Work out the finished part from the listing and answer in its coordinate system (mm). Face numbers are marked on the shaded views. A direction names the side the tool comes from. Coordinates: 2 decimals unless noted, no trailing zeros. Write each loop counter-clockwise with the first axis right and the second up, starting at its lowest first coordinate (ties: lowest second). Pieces come first, ordered by that corner, then holes. Notation, with made-up numbers: M 17.25,73.5 L 76.25,73.5 A8 ccw 76.25,85.5 Z; hole C 80,-20 d11. An arc over 180 degrees is marked long. Answer as CSV lines item,"result". Start each with the question number.
(1) A cutting plane is placed at A-A on y = 28.5. Give the vertices of the cut face in (x, z), then the cut area to 3 significant figures.
(2) Flat-ended cylindrical pins translate along their axes: P1, Ø10, axis at x = -3.5, y = 26.5, coming from the +Z side; P2, Ø10, axis at x = 5, y = 10.5, coming from the -Z side; P3, Ø5, axis at x = 2, y = 31, coming from the -Z side. Find the tip coordinate at first contact, or state that the pin passes through.
(3) The mould has two halves that part along X. Classify the marked faces 1 and 2: released by +X, released by -X, zero draft, split by the parting line, or undercut.
(4) Find the intervals of material crossed by L1, parallel to Y at x = 7, z = -0.5; L2, parallel to Y at x = 5, z = -4.75; L3, parallel to Y at x = -8.5, z = -1.25, in increasing order. Write a range as [from, to].
(5) A cutting plane is placed at B-B on z = -9.5. Give the vertices of the cut face in (x, y), then the cut area to 3 significant figures.
(6) A cutting plane is placed at C-C on y = 8.5. Give the vertices of the cut face in (x, z), then the cut area to 3 significant figures.
(7) For the marked faces 3, 4 and 5, determine the directions among +Z, -Z, +X, -X, +Y, -Y from which every point of the face is accessible in a straight line to the end or side of a thin tool.
from build123d import *
from build123d.topology import SkipClean

# Parameters (mm, degrees)
SKETCH1_R           = 7.5
BOSS_EXTRUDE1_DEPTH = 20
CUT_EXTRUDE2_DEPTH  = 12
CUT_EXTRUDE4_DEPTH  = 1
CHAMFER1_SIZE       = 1
CHAMFER3_SIZE       = 2
CHAMFER4_SIZE       = 1


with BuildPart() as part:
    # Sketch1 → Boss-Extrude1 (new body)
    with BuildSketch(Plane(origin=(0, 0, 0), x_dir=(1, 0, 0), z_dir=(0, 1, 0))):
        with Locations(Location((0, 0, 0), (0, 0, 270))):
            Circle(SKETCH1_R)
    extrude(amount=BOSS_EXTRUDE1_DEPTH)

    # Sketch2 → Revolve1 (revolve)
    with BuildSketch(Plane.XY):
        with BuildLine():
            Line((7.5, 18.99999999999999), (7.5, 20))
            Line((7.5, 20), (0, 20))
            Line((0, 20), (3.1e-16, 39))
            Line((3.1e-16, 39), (7.500000000000009, 39))
            ThreePointArc((7.500000000000009, 39), (12.500000000000009, 28.999999999999993), (7.5, 18.99999999999999))
        make_face()
    revolve(axis=Axis((0, 20, 0), (2e-17, 1, 0)))

    # Sketch3 → Cut-Extrude2 (cut)
    with BuildSketch(Plane(origin=(0, 0, 0), x_dir=(-1, 0, 0), z_dir=(0, -1, 0))):
        with BuildLine():
            Line((-5.099019513592785, -5.5), (0, -5.5))
            Line((0, -5.5), (5.099019513592785, -5.5))
            ThreePointArc((5.099019513592785, -5.5), (-1.21e-15, -7.5), (-5.099019513592785, -5.5))
        make_face()
    extrude(amount=-CUT_EXTRUDE2_DEPTH, mode=Mode.SUBTRACT)

    # Sketch4 → Cut-Extrude4 (cut, symmetric)
    with SkipClean():  # the faces are left unmerged after this step: merging them gives an invalid solid
        with BuildSketch(Plane(origin=(0, 5, 0), x_dir=(1, 0, 0), z_dir=(0, 1, 0))):
            with BuildLine():
                Line((-1.381010726618471, -6.351598961912246), (-1.8059371040395404, -8.305937104039092))
                ThreePointArc((-1.8059371040395404, -8.305937104039092), (-8.451345022667464, 0.9081670043741211), (-2e-17, 8.5))
                ThreePointArc((-2e-17, 8.5), (8.451345022667484, 0.9081670043739513), (1.8059371040392067, -8.305937104039163))
                Line((1.8059371040392067, -8.305937104039163), (1.3810107266181975, -6.351598961912305))
                ThreePointArc((1.3810107266181975, -6.351598961912305), (6.462793252628076, 0.6944806504035996), (1.2e-16, 6.5))
                ThreePointArc((1.2e-16, 6.5), (-6.462793252628061, 0.6944806504037396), (-1.381010726618471, -6.351598961912246))
            make_face()
        extrude(amount=CUT_EXTRUDE4_DEPTH, both=True, mode=Mode.SUBTRACT)

    # Chamfer1
    chamfer1_edges = [part.edges().sort_by_distance(p)[0] for p in [
        (-6.2449979983983965, 6, -1.8027756377319957),
        (6.244997998398398, 4, -1.8027756377319937),
    ]]
    chamfer(chamfer1_edges, length=CHAMFER1_SIZE - 0.0001)  # a hair under: the kernel refuses the full size

    # Chamfer3
    chamfer3_edges = [part.edges().sort_by_distance(p)[0] for p in [
        (0, 12, 5.5),
    ]]
    chamfer(chamfer3_edges, length=CHAMFER3_SIZE - 0.0001)  # a hair under: the kernel refuses the full size

    # Chamfer4
    chamfer4_edges = [part.edges().sort_by_distance(p)[0] for p in [
        (2.3e-15, 0, -7.5),
    ]]
    chamfer(chamfer4_edges, length=CHAMFER4_SIZE)


solid = part.part
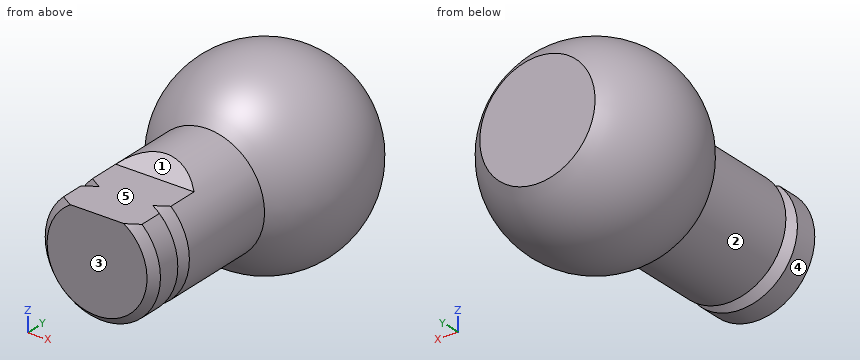
Here are the results:
1,outline,"C 0,0 d24.98"
1,area,"490 mm^2"
2,P1,"stops at z = 12.5"
2,P2,"stops at z = -7.5"
2,P3,"stops at z = -12.5"
3,face 1,"zero draft"
3,face 2,"split by the parting line"
4,L1,"y = [0.52, 4.48], [5.52, 39]"
4,L2,"y = [0.4, 4.6], [5.4, 39]"
4,L3,"y = [19.92, 38.08]"
5,outline,"C 0,29 d16.25"
5,area,"207 mm^2"
6,outline,"M -5.1,5.5 A7.5 ccw long 5.1,5.5 Z"
6,area,"163 mm^2"
7,face 3,"+Z, -Z, +X, -X, -Y"
7,face 4,"-Y"
7,face 5,"+Z, +X, -X, -Y"
